Answer from the drawing. Dimensions are ordinates in mm from the lowest x, y and z of the part. Give positions to 0.01 mm unless a question says otherwise; leave off trailing zeros. Write each loop counter-clockwise with the first axis right and the second up, starting at its lowest first coordinate (ties: lowest second). Pieces come first, ordered by that corner, then holes. Notation, with made-up numbers: M 49,18.5 L 60,18.5 A11 cw 60,38.5 Z; hole C -13.75,-8.75 d7. An arc over 180 degrees is marked long. Answer as a JSON object with one key per item and string values.
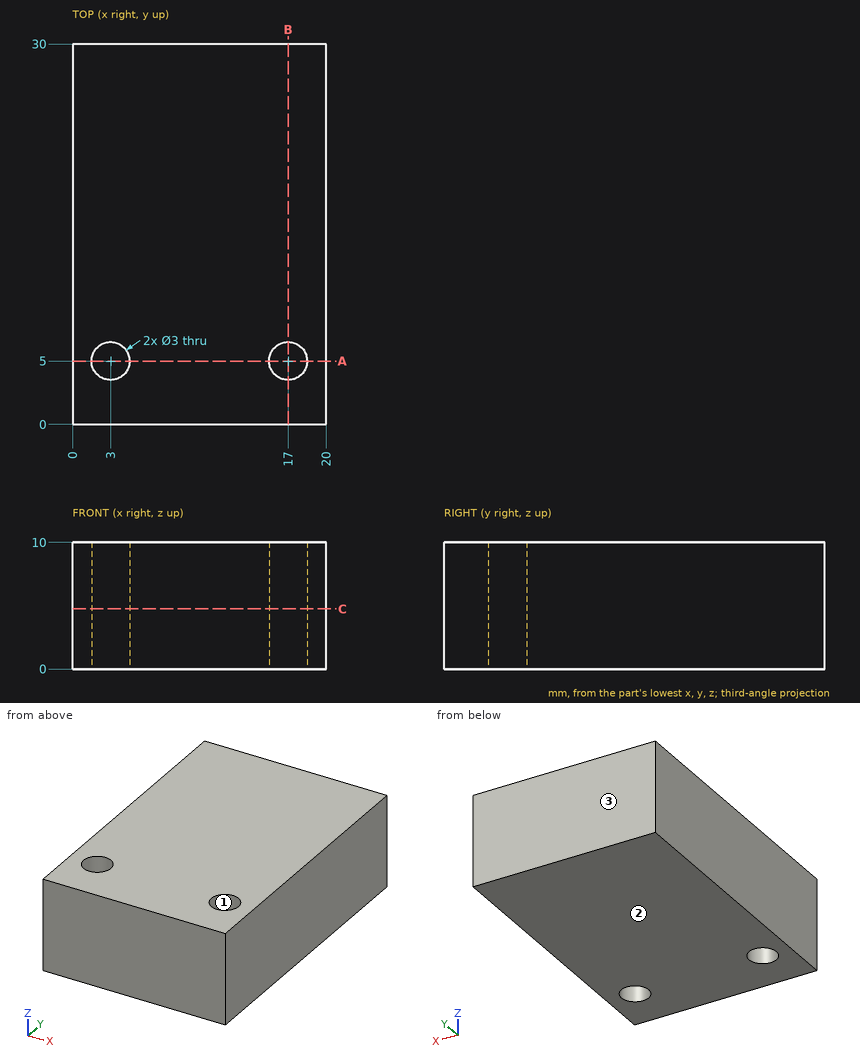
1. A cutting plane is placed at A-A, the plane y = 5. Give the vertices of the cut face in (x, z).
Verdict:
{"outline": "M 0,0 L 1.5,0 L 1.5,10 L 0,10 Z; M 4.5,0 L 15.5,0 L 15.5,10 L 4.5,10 Z; M 18.5,0 L 20,0 L 20,10 L 18.5,10 Z"}
2. A cutting plane is placed at C-C, the plane z = 4.75. Give the vertices of the cut face in (x, y), plus the area to 3 significant figures.
Verdict:
{"outline": "M 0,0 L 20,0 L 20,30 L 0,30 Z; hole C 3,5 d3; hole C 17,5 d3", "area": "586 mm2"}
3. Consider line 1 along X through (y, z) = (5, 4.75); line 2 along Y through (x, z) = (3, 7); line 3 along Y through (x, z) = (18, 7.25). Determine where each line is inside the solid, lowest interval first.
Verdict:
{"line 1": "x = 0 to 1.5, 4.5 to 15.5, 18.5 to 20", "line 2": "y = 0 to 3.5, 6.5 to 30", "line 3": "y = 0 to 3.88, 6.12 to 30"}
4. The mould has two halves that part along Y. Classify the marked faces 1, 2 and 3: released by +Y, released by -Y, zero draft, split by the parting line, or undercut.
Verdict:
{"face 1": "undercut", "face 2": "zero draft", "face 3": "released by +Y"}
5. A cutting plane is placed at B-B, the plane x = 17. Give the vertices of the cut face in (y, z).
Verdict:
{"outline": "M 0,0 L 3.5,0 L 3.5,10 L 0,10 Z; M 6.5,0 L 30,0 L 30,10 L 6.5,10 Z"}
